```python
from build123d import *
from OCP.BRepFilletAPI import BRepFilletAPI_MakeChamfer

# Parameters (mm, degrees)
SKETCH2_R               = 10
BOSS_EXTRUDE1_DEPTH     = 10
SKETCH3_R               = 25
BOSS_EXTRUDE2_DEPTH     = 60
SKETCH4_R               = 30
BOSS_EXTRUDE3_DEPTH     = 5
CHAMFER1_SIZE           = 2.886751346
CHAMFER1_SIZE_2         = 5
CUT_EXTRUDE1_DEPTH      = 82.853527719
CUT_EXTRUDE1_DEPTH_BACK = 82.853527719
SKETCH5_R               = 2.5
SKETCH6_R               = 7.5
BOSS_EXTRUDE4_DEPTH     = 8


with BuildPart() as part:
    # Sketch2 → Boss-Extrude1 (new body)
    with BuildSketch(Plane.XY):
        Circle(SKETCH2_R)
        with BuildLine():
            Line((-1.58113883, 2.25), (1.58113883, 2.25))
            ThreePointArc((1.58113883, 2.25), (0, -2.75), (-1.58113883, 2.25))
        make_face(mode=Mode.SUBTRACT)
    extrude(amount=BOSS_EXTRUDE1_DEPTH)

    # Sketch3 → Boss-Extrude2 (add)
    with BuildSketch(Plane.XY.offset(10)):
        Circle(SKETCH3_R)
    extrude(amount=BOSS_EXTRUDE2_DEPTH)

    # Sketch4 → Boss-Extrude3 (add)
    with BuildSketch(Plane.XY.offset(70)):
        Circle(SKETCH4_R)
    boss_extrude3 = extrude(amount=-BOSS_EXTRUDE3_DEPTH)

    # Mirror1: Boss-Extrude3 across plane
    add(boss_extrude3.mirror(Plane.XY.offset(40)))

    # Chamfer1
    chamfer1_edges_1 = [part.edges().sort_by_distance(p)[0] for p in [
        (-25, 0, 65),
    ]]
    chamfer1_side_1 = [part.faces().sort_by_distance(p)[0] for p in [
        (-25, 0, 64.942264973),
    ]]
    chamfer1_edges_2 = [part.edges().sort_by_distance(p)[0] for p in [
        (-25, 0, 15),
    ]]
    chamfer1_side_2 = [part.faces().sort_by_distance(p)[0] for p in [
        (-25.057735027, 0, 15),
    ]]
    chamfer1 = BRepFilletAPI_MakeChamfer(part.part.solid().wrapped)
    for e in chamfer1_edges_1:
        chamfer1.Add(CHAMFER1_SIZE - 0.0001, CHAMFER1_SIZE_2 - 0.0001, e.wrapped, chamfer1_side_1[0].wrapped)
    for e in chamfer1_edges_2:
        chamfer1.Add(CHAMFER1_SIZE_2 - 0.0001, CHAMFER1_SIZE - 0.0001, e.wrapped, chamfer1_side_2[0].wrapped)
    add(Compound.cast(chamfer1.Shape()), mode=Mode.REPLACE)  # a hair under: the kernel refuses the full size

    # Sketch5 → Cut-Extrude1 (cut, two sides: drawn at the far end of the back side and taken through both)
    with BuildSketch(Plane(origin=(0, 0, 0), x_dir=(0, 0, -1), z_dir=(1, 0, 0)).offset(-CUT_EXTRUDE1_DEPTH_BACK)):
        with Locations((-40, 0)):
            Circle(SKETCH5_R)
    extrude(amount=CUT_EXTRUDE1_DEPTH + CUT_EXTRUDE1_DEPTH_BACK, mode=Mode.SUBTRACT)

    # Sketch6 → Boss-Extrude4 (add)
    with BuildSketch(Plane.XY.offset(70)):
        Circle(SKETCH6_R)
    extrude(amount=BOSS_EXTRUDE4_DEPTH)


solid = part.part
```
Source: CAD feature listing. Evaluate the final solid. Frame: model axes, mm. A direction names the side the tool comes from. Coordinates: 2 decimals unless noted, no trailing zeros. Order: outer loops, then holes, each group sorted by start corner. A loop starts at its lowest first (then second) coordinate and runs counter-clockwise, first axis right, second up. Notation, with made-up numbers: (23, 85.25) - (67, 85.25) arc R20 ccw to (67, 113.25) - close; hole circle Ø1 at (25.5, -14.75). An arc over 180 degrees is marked (long way). One line per item, written item: value.
1) Cut plane D-D on z = 40. Output: boundary loops of the cut face in (x, y).
Computed values:
outline: (-24.87, -2.5) arc R25 ccw to (24.87, -2.5) - close; (-24.87, 2.5) - (24.87, 2.5) arc R25 ccw to start
2) Ray query, line 1 (Y direction, x = 0, z = 5); line 2 (Z direction, x = 1, y = 14.5); line 3 (Y direction, x = 11, z = 40). Return the intervals inside material, ascending. Write a range as [from, to].
Computed values:
line 1: y = [-10, -2.75], [2.25, 10]
line 2: z = [10, 70]
line 3: y = [-22.45, -2.5], [2.5, 22.45]
3) Reachability of faces 4 (the face through (2.1, -2.1, 0)), 5 (the face through (6, -6, 70)), 6 (the face through (-29.97, 1.32, 67.54)), 7 (the face through (-5.487, 24.711, 62.294)), 8 (the face through (0.1, -2.75, 4.93)) from +Z, -Z, +X, -X, +Y, -Y: full face, straight path, thin tool, end or side. Return the list, or none.
Computed values:
face 4: -Z, +X, -X, +Y, -Y
face 5: +Z
face 6: +Z, -Z
face 7: none
face 8: -Z
4) Contact query for flat-ended pins moving along their axis: pin 1 (4 mm diameter, centred on y = -15, z = 22, fed in from -X); pin 2 (12 mm diameter, centred on y = -1, z = 33, fed in from -X); pin 3 (1.5 mm diameter, centred on x = 20.5, y = 5, fed in from +Z). Output: stop coordinate, or through.
Computed values:
pin 1: stops at x = -21.35
pin 2: stops at x = -25
pin 3: stops at z = 70
5) Mould query, pull axis Y, two halves, no side actions, for faces 1 (the face through (23.846, 7.509, 39.69)), 2 (the face through (-0.35, -0.96, 37.69)), 3 (the face through (13, 0, 10)). Classes: released by +Y, released by -Y, zero draft, split by the parting line, or undercut.
Computed values:
face 1: split by the parting line
face 2: undercut
face 3: zero draft
6) Cut plane C-C on z = 5. Output: boundary loops of the cut face in (x, y), plus the area to 3 significant figures.
Computed values:
outline: circle Ø20 at (0, 0); hole (-1.58, 2.25) arc R2.75 ccw (long way) to (1.58, 2.25) - close
area: 291 mm^2
